The figure shows three views and two pictorial views of one solid part (mm, origin at its lowest corner). Answer the questions. A direction names the side the tool comes from. Coordinates: 2 decimals unless noted, no trailing zeros. Write each loop counter-clockwise with the first axis right and the second up, starting at its lowest first coordinate (ties: lowest second). Pieces come first, ordered by that corner, then holes. Notation, with made-up numbers: (66, -30.5) -> (120, -30.5) arc R33 cw to (120, 0.5) -> close; hole circle Ø9 at (82.5, -38.75). An arc over 180 degrees is marked (long way). Use CSV: the item, a comma, the result in double quotes. Start each with the question number.
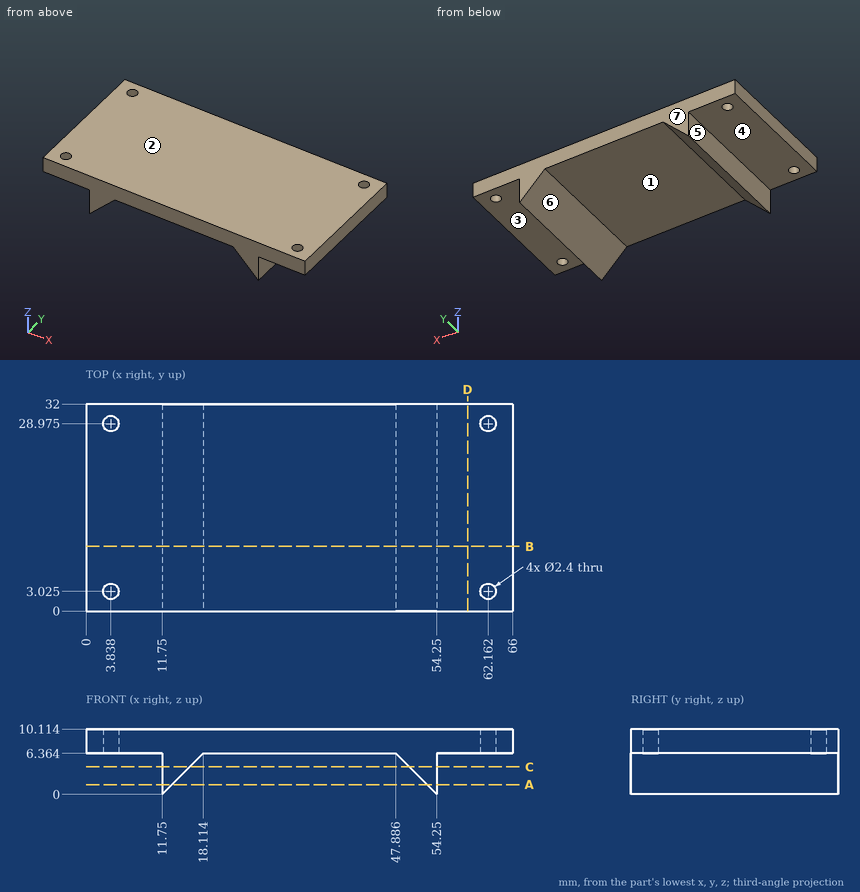
1) Each of these flat-tipped pins is pushed along its axis until it touches: pin 1 (3 mm diameter, centred on x = 48.5, z = 2.5, fed in from -Y); pin 2 (1.9 mm diameter, centred on y = 12.5, z = 3.5, fed in from -X); pin 3 (6 mm diameter, centred on x = 34.5, y = 27, fed in from -Z); pin 4 (13 mm diameter, centred on x = 58.5, y = 14, fed in from -Z). Where does it stop, or does it pass through?
2) Find the intervals of material crossed by line 1 along Z through (x, y) = (57.5, 24); line 2 along Y through (x, z) = (61.5, 6.5) (1 decimal); line 3 along X through (y, z) = (12.5, 3.75), in increasing order.
3) Section C-C, the plane z = 4.25 is taken. Give the vertices of the cut face in (x, y), plus the area to 3 significant figures.
4) Section B-B, the plane y = 10 is taken. Give the vertices of the cut face in (x, z), plus the area to 3 significant figures.
5) The mould has two halves that part along X. Classify the marked faces 5, 6 and 7: pulls with the +X half, pulls with the -X half, needs draft (parallel to the pull), parting line crosses it, or undercut.
6) Which of the six approach directions +Z, -Z, +X, -X, +Y, -Y give full straight-line access (tool end or side, diameter ignored) to the marked faces 1, 2, 3 and 4?
7) Section D-D, the plane x = 59 is taken. Give the vertices of the cut face in (y, z).
8) Section A-A, the plane z = 1.5 is taken. Give the vertices of the cut face in (x, y).
The answers:
1,pin 1,"passes through"
1,pin 2,"stops at x = 11.75"
1,pin 3,"stops at z = 6.36"
1,pin 4,"stops at z = 0"
2,line 1,"z = 6.36 to 10.11"
2,line 2,"y = 0 to 2, 4 to 28, 30 to 32"
2,line 3,"x = 11.75 to 15.5, 50.5 to 54.25"
3,outline,"(11.75, 0) -> (16, 0) -> (16, 32) -> (11.75, 32) -> close; (50, 0) -> (54.25, 0) -> (54.25, 32) -> (50, 32) -> close"
3,area,"272 mm^2"
4,outline,"(0, 6.36) -> (11.75, 6.36) -> (11.75, 0) -> (18.11, 6.36) -> (47.89, 6.36) -> (54.25, 0) -> (54.25, 6.36) -> (66, 6.36) -> (66, 10.11) -> (0, 10.11) -> close"
4,area,"288 mm^2"
5,face 5,"pulls with the -X half"
5,face 6,"undercut"
5,face 7,"needs draft"
6,face 1,"-Z, +Y, -Y"
6,face 2,"+Z, +X, -X, +Y, -Y"
6,face 3,"-Z, +X, +Y, -Y"
6,face 4,"-Z, -X, +Y, -Y"
7,outline,"(0, 6.36) -> (32, 6.36) -> (32, 10.11) -> (0, 10.11) -> close"
8,outline,"(11.75, 0) -> (13.25, 0) -> (13.25, 32) -> (11.75, 32) -> close; (52.75, 0) -> (54.25, 0) -> (54.25, 32) -> (52.75, 32) -> close"
